Autodesk Inventor part; units mm, degrees
ref_plane "YZ Plane" through (0, 0, 0) normal (1, 0, 0) x (0, 1, 0)
ref_plane "XZ Plane" through (0, 0, 0) normal (0, 1, 0) x (-1, 0, 0)
ref_plane "XY Plane" through (0, 0, 0) normal (0, 0, 1) x (1, 0, 0)
sketch "Sketch1" plane through (0, 0, 0) normal (0, 1, 0) x (-1, 0, 0)
  line L0 (-666.6265, 392.3922) -> (-666.6265, -14.0078)
  line L1 (6.4735, -14.0078) -> (6.4735, 392.3922)
  line L2 (-196.7265, 392.3922) -> (-196.7265, 525.7422)
  line L3 (-196.7265, 525.7422) -> (-463.4265, 525.7422)
  line L4 (-463.4265, 525.7422) -> (-463.4265, 392.3922)
  line L5 (6.4735, 392.3922) -> (-196.7265, 392.3922)
  line L6 (-463.4265, 392.3922) -> (-666.6265, 392.3922)
  line L7 (-196.7265, -14.0078) -> (-196.7265, -147.3578)
  line L8 (-196.7265, -147.3578) -> (-463.4265, -147.3578)
  line L9 (-463.4265, -147.3578) -> (-463.4265, -14.0078)
  line L10 (-666.6265, -14.0078) -> (-463.4265, -14.0078)
  line L11 (-196.7265, -14.0078) -> (6.4735, -14.0078)
  point P0 (0, 0)
  dimension "d0" = 673.1
  dimension "d1" = 406.4
  dimension "d73" = 266.7
  dimension "d75" = 203.2
  dimension "d76" = 266.7
extrude "Extrusion1" add sketch "Sketch1" along normal blind 6.35
sketch "Sketch2" plane through (0, 6.35, 0) normal (0, 1, 0) x (1, 0, 0)
  line L0 (666.6265, -392.3922) -> (666.6265, 14.0078)
  line L1 (666.6265, -392.3922) -> (666.6265, -290.7922)
  line L2 (666.6265, -290.7922) -> (666.6265, -189.1922) construction
  line L3 (666.6265, 14.0078) -> (666.6265, -58.7236) construction
  line L4 (666.6265, 14.0078) -> (666.6265, -87.5922) construction
  line L5 (-6.4735, 14.0078) -> (-6.4735, -392.3922) construction
  line L6 (-6.4735, -392.3922) -> (241.1765, -392.3922) construction
  line L7 (-6.4735, -392.3922) -> (666.6265, -392.3922) construction
  line L8 (666.6265, -392.3922) -> (418.9765, -392.3922) construction
  circle A0 centre (653.9265, -290.7922) radius 3.175
  circle A1 centre (653.9265, -87.5922) radius 3.175
  circle A2 centre (241.1765, -379.6922) radius 3.175
  circle A3 centre (418.9765, -379.6922) radius 3.175
  circle A4 centre (418.9765, 1.3078) radius 3.175
  circle A5 centre (241.1765, 1.3078) radius 3.175
  circle A6 centre (6.2265, -87.5922) radius 3.175
  circle A7 centre (6.2265, -290.7922) radius 3.175
  circle A8 centre (6.2265, -239.9922) radius 3.9751
  circle A9 centre (6.2265, -138.3922) radius 3.9751
  circle A10 centre (653.9265, -239.9922) radius 3.9751
  circle A11 centre (653.9265, -138.3922) radius 3.9751
  line L9 (458.3979, 14.0078) -> (460.8865, 14.0078)
  line L10 (460.8865, 14.0078) -> (460.8865, -3.7722)
  line L11 (460.8865, -3.7722) -> (448.1865, -3.7722)
  line L12 (448.1865, -3.7722) -> (448.1865, 7.197)
  line L13 (448.1865, 7.197) -> (460.8865, 7.197)
  line L14 (460.8865, 7.197) -> (460.8865, -3.7722)
  line L15 (666.6265, 14.0078) -> (-6.4735, 14.0078)
  circle A12 centre (330.0765, -513.0422) radius 3.9751
  line L16 (196.7265, -392.3922) -> (196.7265, -525.7422)
  circle A13 centre (330.0765, 134.6578) radius 3.9751
  line L17 (196.7265, 147.3578) -> (196.7265, 14.0078)
  line L18 (196.7265, -525.7422) -> (463.4265, -525.7422)
  line L19 (463.4265, 147.3578) -> (196.7265, 147.3578)
  point P0 (0, 0)
  dimension "d11" = 6.35
  dimension "d12" = 6.35
  dimension "d13" = 12.7
  dimension "d14" = 12.7
  dimension "d15" = 6.35
  dimension "d16" = 12.7
  dimension "d17" = 6.35
  dimension "d18" = 12.7
  dimension "d19" = 6.35
  dimension "d20" = 6.35
  dimension "d23" = 6.35
  dimension "d24" = 6.35
  dimension "d25" = 12.7
  dimension "d26" = 12.7
  dimension "d34" = 7.9502
  dimension "d35" = 7.9502
  dimension "d40" = 50.8
  dimension "d43" = 50.8
  dimension "d44" = 7.9502
  dimension "d45" = 7.9502
  dimension "d46" = 50.8
  dimension "d66" = 205.74
  dimension "d68" = 12.7
  dimension "d70" = 17.78
  dimension "d78" = 7.9502
  dimension "d79" = 133.35
  dimension "d80" = 7.9502
  dimension "d81" = 133.35
  dimension "d82" = 12.7
  dimension "d83" = 12.7
hole "Hole1" at (653.9265, 6.35, 290.7922) at (653.9265, 6.35, 87.5922) at (418.9765, 6.35, -1.3078) at (241.1765, 6.35, -1.3078) at (418.9765, 6.35, 379.6922) at (241.1765, 6.35, 379.6922) at (6.2265, 6.35, 290.7922) at (6.2265, 6.35, 87.5922) at (6.2265, 6.35, 239.9922) at (6.2265, 6.35, 138.3922) at (653.9265, 6.35, 239.9922) at (653.9265, 6.35, 138.3922) at (330.0765, 6.35, 513.0422) at (330.0765, 6.35, -134.6578) direction (0, -1, 0) diameter 7.9502 end through all
sketch "Sketch3" plane through (0, 6.35, 0) normal (0, 1, 0) x (1, 0, 0)
  line L0 (-6.4735, -392.3922) -> (666.6265, -392.3922)
  line L1 (-6.4735, -392.3922) -> (63.1225, -392.3922)
  line L2 (63.1225, -392.3922) -> (63.1225, -366.9922)
  line L3 (63.1225, -366.9922) -> (18.9265, -366.9922)
  line L4 (-6.4735, -366.9922) -> (-6.4735, -392.3922)
  line L5 (-6.4735, -392.3922) -> (18.9265, -392.3922)
  line L6 (18.9265, -366.9922) -> (18.9265, -322.7962)
  line L7 (18.9265, -322.7962) -> (-6.4735, -322.7962)
  line L8 (-6.4735, -322.7962) -> (-6.4735, -392.3922)
  line L9 (666.6265, 14.0078) -> (-6.4735, 14.0078)
  line L10 (-6.4735, 14.0078) -> (63.1225, 14.0078)
  line L11 (63.1225, 14.0078) -> (63.1225, -11.3922)
  line L12 (63.1225, -11.3922) -> (18.9265, -11.3922)
  line L13 (-6.4735, -11.3922) -> (-6.4735, 14.0078)
  line L14 (-6.4735, 14.0078) -> (18.9265, 14.0078)
  line L15 (18.9265, -11.3922) -> (18.9265, -55.5882)
  line L16 (18.9265, -55.5882) -> (-6.4735, -55.5882)
  line L17 (-6.4735, -55.5882) -> (-6.4735, 14.0078)
  line L18 (666.6265, -392.3922) -> (641.2265, -392.3922)
  line L19 (641.2265, -366.9922) -> (641.2265, -322.7962)
  line L20 (641.2265, -322.7962) -> (666.6265, -322.7962)
  line L21 (666.6265, -322.7962) -> (666.6265, -392.3922)
  line L22 (666.6265, -392.3922) -> (597.0305, -392.3922)
  line L23 (597.0305, -392.3922) -> (597.0305, -366.9922)
  line L24 (597.0305, -366.9922) -> (641.2265, -366.9922)
  line L25 (666.6265, -366.9922) -> (666.6265, -392.3922)
  line L26 (666.6265, 14.0078) -> (597.0305, 14.0078)
  line L27 (597.0305, 14.0078) -> (597.0305, -11.3922)
  line L28 (597.0305, -11.3922) -> (641.2265, -11.3922)
  line L29 (666.6265, -11.3922) -> (666.6265, 14.0078)
  line L30 (666.6265, 14.0078) -> (641.2265, 14.0078)
  line L31 (641.2265, -11.3922) -> (641.2265, -55.5882)
  line L32 (641.2265, -55.5882) -> (666.6265, -55.5882)
  line L33 (666.6265, -55.5882) -> (666.6265, 14.0078)
  point P0 (0, 0)
  dimension "d47" = 69.596
  dimension "d48" = 25.4
  dimension "d49" = 25.4
  dimension "d50" = 69.596
  dimension "d51" = 69.596
  dimension "d52" = 25.4
  dimension "d53" = 25.4
  dimension "d54" = 69.596
  dimension "d55" = 25.4
  dimension "d56" = 69.596
  dimension "d57" = 69.596
  dimension "d58" = 25.4
  dimension "d59" = 69.596
  dimension "d60" = 25.4
  dimension "d61" = 25.4
  dimension "d62" = 69.596
extrude "Extrusion2" cut sketch "Sketch3" against normal blind 25.4
sketch "Sketch4" plane through (0, 6.35, 0) normal (0, 1, 0) x (1, 0, 0)
  line L0 (-6.4735, -55.5882) -> (-6.4735, -322.7962) construction
  line L1 (666.6265, -322.7962) -> (666.6265, -55.5882) construction
  point P0 (0, 0)
properties part number "Polyc_for_swerve" material "Polycarbonate, Clear"
CAD build for the part. Positions are in the model's coordinates, mm. Round coordinates to 2 decimals unless told otherwise and drop trailing zeros. Write each loop counter-clockwise with the first axis right and the second up, starting at its lowest first coordinate (ties: lowest second). Pieces come first, ordered by that corner, then holes. Notation, with made-up numbers: M 40.5,-28 L 67.5,-28 A11 cw 67.5,-16 Z; hole C 67,52.25 d6. An arc over 180 degrees is marked long. Use a Markdown table: item, result. Add a question column.
1. Drill centre lines: probe 1 along X at (y, z) = (6, 239); probe 2 along Z at (x, y) = (333, 2.75); probe 3 along Z at (x, y) = (328, 1). Where is each one in solid material? Low to high.
2. Flat gauge pins, fed straight in: P1, Ø1.9, axis at y = 4.5, z = 39.5, coming from the +X side; P2, Ø3, axis at x = 654, y = 4, coming from the -Z side; P3, Ø1.5, axis at x = 511.5, y = 3.5, coming from the -Z side. Where does each tip first touch, or does it go through?
3. Pull direction Y, two halves, no side cores. Call faces 1 (the face through (335, 6.35, 194)), 2 (the face through (335, 0, 194)): released by +Y, released by -Y, zero draft, split by the parting line, or undercut.
4. Slice it at C-C on y = 5. Give the number of separate pieces and of enclosed holes in the cut face, then the cut area to 3 significant figures.
5. Slice it at B-B on x = 566. Give the cut face in (y, z).
6. Slice it at A-A on z = 41.5. Give the cut face in (x, y), then the cut area to 3 significant figures.
Reply:
| question | item | result |
|---|---|---|
| 1 | probe 1 | x = -6.47 to 2.38, 10.08 to 650.08, 657.78 to 666.63 |
| 1 | probe 2 | z = -147.36 to -137.35, -131.96 to 510.35, 515.74 to 525.74 |
| 1 | probe 3 | z = -147.36 to -138.05, -131.27 to 509.65, 516.43 to 525.74 |
| 2 | P1 | stops at x = 641.23 |
| 2 | P2 | stops at z = 55.59 |
| 2 | P3 | stops at z = -14.01 |
| 3 | face 1 | released by +Y |
| 3 | face 2 | released by -Y |
| 4 | separate pieces | 1 |
| 4 | enclosed holes | 14 |
| 4 | area | 332,000 mm^2 |
| 5 | outline | M 0,-14.01 L 6.35,-14.01 L 6.35,392.39 L 0,392.39 Z |
| 6 | outline | M 18.93,0 L 641.23,0 L 641.23,6.35 L 18.93,6.35 Z |
| 6 | area | 3,950 mm^2 |
